from build123d import *

# Parameters (mm, degrees)
F0_R      = 22.225
F1_DEPTH  = 50.8
F2_R      = 4.7625
F3_DEPTH  = 3.048
F4_R      = 1.5875
F5_DEPTH  = 16.002
F7_DEPTH  = 10.16
F8_R      = 5.08
F9_W      = 7.874
F9_H      = 60.452
F10_DEPTH = 3.302
F11_R     = 1.9812
F12_DEPTH = 50.801


with BuildPart() as f1:
    # F0 (on Front) → F1 (new body)
    with BuildSketch(Plane.XZ):
        Circle(F0_R)
    extrude(amount=F1_DEPTH)

    # F2 (on face) → F3 (join)
    with BuildSketch(Plane.XZ.offset(50.8)):
        Circle(F2_R)
    extrude(amount=F3_DEPTH)

    # F4 (on face) → F5 (join)
    with BuildSketch(Plane.XZ.offset(53.848)):
        Circle(F4_R)
    extrude(amount=F5_DEPTH)

    # F6 (on face) → F7 (cut)
    with BuildSketch(Plane.XZ.offset(69.85)):
        with BuildLine():
            Line((-0.9525, -1.27), (-0.9525, 1.27))
            ThreePointArc((-0.9525, 1.27), (-1.5875, 0), (-0.9525, -1.27))
        make_face()
    extrude(amount=-F7_DEPTH, mode=Mode.SUBTRACT)

    # F8
    f8_edges = [f1.edges().sort_by_distance(p)[0] for p in [
        (-22.225, 0, 0),
    ]]
    fillet(f8_edges, radius=F8_R)

    # F9 (on face) → F10 (join)
    with BuildSketch(Plane.XZ.offset(50.8)):
        Rectangle(F9_W, F9_H)
    extrude(amount=-F10_DEPTH)

    # F11 (on face) → F12 (cut, through all)
    with BuildSketch(Plane.XZ.offset(50.8)):
        with Locations((0, 26.035)):
            Circle(F11_R)
        with Locations((0, -26.035)):
            Circle(F11_R)
    extrude(amount=-F12_DEPTH, mode=Mode.SUBTRACT)


solid = f1.part
The model under review builds one solid part; all positions refer to its coordinate system, in mm. A direction names the side the tool comes from. Round coordinates to 2 decimals unless told otherwise and drop trailing zeros. Loops run counter-clockwise (first coordinate to the right, second up) from the corner with the lowest first, then second, coordinate; pieces in that order, holes last. Notation, with made-up numbers: (3, 86.25) -> (28, 86.25) arc R25 ccw to (28, 120.25) -> close; hole circle Ø8 at (3.25, 11). An arc over 180 degrees is marked (long way). Answer as CSV lines item,"result".
1) Add section C-C on z = 25. Write out the cut boundary in (x, y), plus the area to 3 significant figures.
Geometry results:
outline,"(-3.94, -50.8) -> (-1.69, -50.8) -> (-1.69, -47.5) -> (-3.94, -47.5) -> close; (1.69, -50.8) -> (3.94, -50.8) -> (3.94, -47.5) -> (1.69, -47.5) -> close"
area,"14.8 mm²"
2) Draft analysis for pull direction Z (two halves, no side actions). For faces 4 (the face through (3.937, -49, 26)), 5 (the face through (-0.26, -49.17, 28)), 6 (the face through (1.514, -61.737, 0.477)), state which applies: pulls with the +Z half, pulls with the -Z half, needs draft (parallel to the pull), parting line crosses it, or undercut.
Geometry results:
face 4,"needs draft"
face 5,"undercut"
face 6,"parting line crosses it"
3) Tool access review of faces 1 (the face through (-3.937, -49, 26)), 2 (the face through (-3.78, -52.3, -2.9)), 3 (the face through (3.937, -49, -26)): name each direction out of +Z, -Z, +X, -X, +Y, -Y from which nothing blocks a thin tool from reaching the whole face with its end or side.
Geometry results:
face 1,"+Z, -X, +Y, -Y"
face 2,"-Y"
face 3,"-Z, +X, +Y, -Y"
4) Add section A-A on x = 0. State how many separate pieces and enclosed holes the cut face has, plus the area to 3 significant figures.
Geometry results:
separate pieces,"3"
enclosed holes,"0"
area,"2,350 mm²"
5) To check wall thickness, follow line 1 along Z through (x, y) = (0, -49); line 2 along Z through (x, y) = (0, -36) (3 decimals); line 3 along Y through (x, z) = (-4, -8). State the ranges of each line that lie inside material, in increasing order. Write a range as from..to.
Geometry results:
line 1,"z = -30.23..-28.02, -24.05..24.05, 28.02..30.23"
line 2,"z = -22.225..22.225"
line 3,"y = -50.8..0"
6) Add section D-D on y = -61.5. Write out the cut boundary in (x, z) (1 decimal).
Geometry results:
outline,"(-1, -1.3) arc R1.6 ccw (long way) to (-1, 1.3) -> close"
7) For P1, Ø2, axis at y = -65, z = 0, coming from the -X side; P2, Ø1, axis at x = -9.5, y = -34.5, coming from the +Z side; P3, Ø12, axis at x = -5, y = -25, coming from the +Z side (3 decimals); P4, Ø1.5, axis at x = -6.5, y = -54.5, coming from the -Z side, all flat-tipped, find the tip position at first contact; note any pin that passes through.
Geometry results:
P1,"stops at x = -0.95"
P2,"stops at z = 20.32"
P3,"stops at z = 22.225"
P4,"passes through"
